Verification items for the finished model (mm, model axes). Coordinates: 2 decimals unless noted, no trailing zeros. Order: outer loops, then holes, each group sorted by start corner. A loop starts at its lowest first (then second) coordinate and runs counter-clockwise, first axis right, second up.
Q1. Cross-section at B-B, the plane y = 19.05. Record the boundary of the cut face in (x, z).
Q2. Cross-section at A-A, the plane x = 127. Record the boundary of the cut face in (y, z) (1 decimal), and give its area (3 significant figures).
Q3. Cross-section at C-C, the plane z = 1.2. Count the separate pieces of the cut face and the enclosed holes in it, and give its area (3 significant figures).
Q4. Thickness scan on line 1 (Y direction, x = 101.6, z = 0.7) (3 decimals); line 2 (X direction, y = 5, z = 0.55); line 3 (X direction, y = 15.5, z = 0.85). Record the ranges inside material, lowest first.
Q5. Cross-section at D-D, the plane x = 101.6. Record the boundary of the cut face in (y, z) (1 decimal), and give its area (3 significant figures).
Q6. Draft check along Y on faces 1 (the cylindrical face through (53.223, 11.937, 0.783)), 2 (the flat face through (69, 21, 1.588)). Enter one of: pulls with the +Y half, pulls with the -Y half, needs draft (parallel to the pull), parting line crosses it, or undercut.
Autodesk Inventor part; units mm, degrees
ref_plane "YZ Plane" through (0, 0, 0) normal (1, 0, 0) x (0, 1, 0)
ref_plane "XZ Plane" through (0, 0, 0) normal (0, 1, 0) x (-1, 0, 0)
ref_plane "XY Plane" through (0, 0, 0) normal (0, 0, 1) x (1, 0, 0)
sketch "Sketch1" plane through (0, 0, 0) normal (0, 0, 1) x (1, 0, 0)
  line L0 (0, 0) -> (139.7, 0)
  line L1 (139.7, 0) -> (139.7, 41.275)
  line L2 (139.7, 41.275) -> (0, 41.275)
  line L3 (0, 41.275) -> (0, 0)
  circle A0 centre (12.7, 12.7) radius 2.54
  circle A1 centre (25.4, 12.7) radius 4.445
  circle A2 centre (38.1, 12.7) radius 2.54
  circle A3 centre (50.8, 12.7) radius 2.54
  circle A4 centre (76.2, 12.7) radius 2.54
  circle A5 centre (88.9, 12.7) radius 4.445
  circle A6 centre (101.6, 12.7) radius 2.54
  circle A7 centre (127, 12.7) radius 4.445
  circle A8 centre (133.35, 19.05) radius 2.54
  circle A9 centre (133.35, 6.35) radius 2.54
  circle A10 centre (120.65, 6.35) radius 2.54
  circle A11 centre (120.65, 19.05) radius 2.54
  circle A12 centre (6.35, 34.925) radius 2.54
  dimension "d0" = 139.7
  dimension "d1" = 41.275
  dimension "d6" = 5.08
  dimension "d12" = 8.89
  dimension "d13" = 5.08
  dimension "d14" = 5.08
  dimension "d15" = 5.08
  dimension "d19" = 8.89
  dimension "d20" = 5.08
  dimension "d21" = 8.89
  dimension "d24" = 5.08
  dimension "d28" = 5.08
  dimension "d29" = 5.08
  dimension "d30" = 5.08
  dimension "d34" = 5.08
extrude "Extrusion1" add sketch "Sketch1" along normal blind 1.5875
properties part number "flatPoly1ForCNC"
Check values:
1. outline: (0, 0) - (118.11, 0) - (118.11, 1.59) - (0, 1.59) - close; (123.19, 0) - (130.81, 0) - (130.81, 1.59) - (123.19, 1.59) - close; (135.89, 0) - (139.7, 0) - (139.7, 1.59) - (135.89, 1.59) - close
2. outline: (0, 0) - (8.3, 0) - (8.3, 1.6) - (0, 1.6) - close; (17.1, 0) - (41.3, 0) - (41.3, 1.6) - (17.1, 1.6) - close
2. area: 51.4 mm2
3. separate pieces: 1
3. enclosed holes: 13
3. area: 5,380 mm2
4. line 1: y = 0 to 10.16, 15.24 to 41.275
4. line 2: x = 0 to 118.5, 122.8 to 131.2, 135.5 to 139.7
4. line 3: x = 0 to 21.95, 28.85 to 85.45, 92.35 to 123.55, 130.45 to 139.7
5. outline: (0, 0) - (10.2, 0) - (10.2, 1.6) - (0, 1.6) - close; (15.2, 0) - (41.3, 0) - (41.3, 1.6) - (15.2, 1.6) - close
5. area: 57.5 mm2
6. face 1: undercut
6. face 2: needs draft
